Design review of the part shown in the three views and the two pictorial views. Dimensions are in mm from the part's minimum x, y and z. A direction names the side the tool comes from. Round coordinates to 2 decimals unless told otherwise and drop trailing zeros. Order: outer loops, then holes, each group sorted by start corner. A loop starts at its lowest first (then second) coordinate and runs counter-clockwise, first axis right, second up. Notation, with made-up numbers: M -12,-24.75 L 0,-24.75 A10 cw 0,-14.75 Z; hole C 74.5,26 d1. An arc over 180 degrees is marked long. Write each question's results on one line, items separated by ' | '. Start each with the question number.
Item 1: Machinability: for the marked faces 1, 2, 3, 4 and 5, which of the approach directions +Z, -Z, +X, -X, +Y, -Y give a long, thin tool a straight path to every point of the face, cutting with its end or side? Answer none if there is none.
Item 2: Take a section at D-D, the plane y = 27.5. Write out the cut boundary in (x, z).
Item 3: Take a section at B-B, the plane y = 13.5. Write out the cut boundary in (x, z), plus the area to 3 significant figures.
Item 4: Take a section at C-C, the plane z = 15. Write out the cut boundary in (x, y), plus the area to 3 significant figures.
Item 5: Take a section at A-A, the plane x = 17.5. Write out the cut boundary in (y, z).
Item 6: Wall thickness on line 1 (X direction, y = 24.5, z = 32.5); line 2 (X direction, y = 35, z = 17.5); line 3 (Z direction, x = 30.5, y = 19.5): over which ranges is each line inside the solid? List them lowest first. Write a range as [from, to].
Item 7: Clearance check with flat-ended pins moving along their axes: pin 1 (22 mm diameter, centred on y = 9.5, z = 29, fed in from -X); pin 2 (22 mm diameter, centred on y = 29.5, z = 26.5, fed in from -X); pin 3 (2 mm diameter, centred on x = 31, y = 7.5, fed in from -Z); pin 4 (5 mm diameter, centred on x = 5.5, y = 12, fed in from +Z). State where each tip first meets the part, or that it passes through.
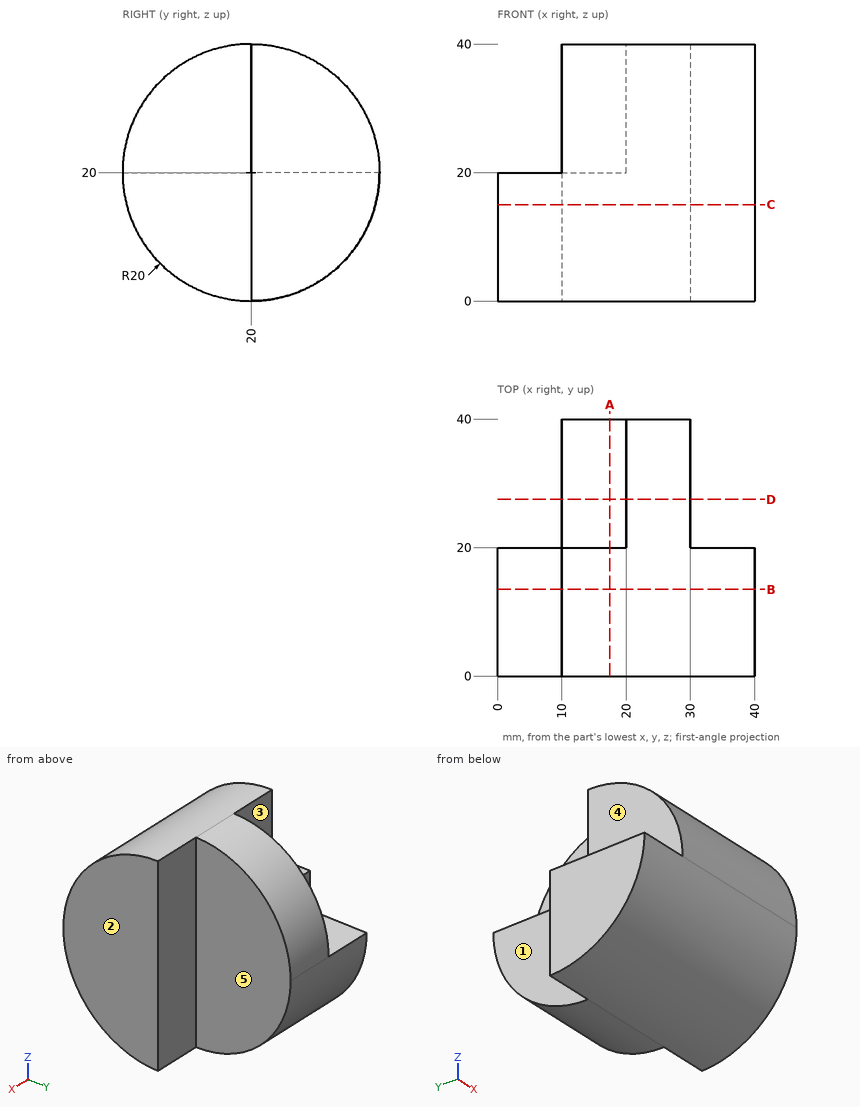
Results list:
1) face 1: +Z, -Z, -X, +Y | face 2: +Z, -Z, +X, +Y, -Y | face 3: +Z, -X, +Y | face 4: +Z, -X, +Y, -Y | face 5: +Z, -Z, +X, +Y
2) outline: M 10,1.46 L 30,1.46 L 30,38.54 L 20,38.54 L 20,20 L 10,20 Z
3) outline: M 0,1.09 L 40,1.09 L 40,38.91 L 10,38.91 L 10,20 L 0,20 Z | area: 1,320 mm²
4) outline: M 0,0.64 L 40,0.64 L 40,20 L 30,20 L 30,39.36 L 10,39.36 L 10,20 L 0,20 Z | area: 1,160 mm²
5) outline: M 20,20 L 20,40 A20 ccw long 40,20 Z
6) line 1: [20, 30] | line 2: [10, 30] | line 3: [0.01, 39.99]
7) pin 1: x = 0 | pin 2: x = 10 | pin 3: z = 3.64 | pin 4: z = 20
